```python
from build123d import *

# Parameters (mm, degrees)
F0_R     = 2.89
F0_R_2   = 2.35
F1_DEPTH = 0.81
F0_R_3   = 1.85
F2_DEPTH = 7.885
F3_DEPTH = 0.05


with BuildPart() as f1:
    # F0 (on Front) → F1 (new body, symmetric)
    with BuildSketch(Plane.XZ):
        Circle(F0_R)
        Circle(F0_R_2, mode=Mode.SUBTRACT)
    extrude(amount=F1_DEPTH, both=True)

    # F0 (on Front) → F2 (join, symmetric)
    with BuildSketch(Plane.XZ):
        Circle(F0_R_2)
        Circle(F0_R_3, mode=Mode.SUBTRACT)
    extrude(amount=F2_DEPTH, both=True)

    # F0 (on Front) → F3 (join, symmetric)
    with BuildSketch(Plane.XZ):
        Circle(F0_R_3)
    extrude(amount=F3_DEPTH, both=True)


solid = f1.part
```
Geometry: final body of the model. Coordinates: model frame, mm. A direction names the side the tool comes from. Coordinates: 2 decimals unless noted, no trailing zeros. Write each loop counter-clockwise with the first axis right and the second up, starting at its lowest first coordinate (ties: lowest second). Pieces come first, ordered by that corner, then holes. Notation, with made-up numbers: M 4.5,41 L 48.5,41 A23 cw 48.5,73 Z; hole C 68.5,-24.5 d3. An arc over 180 degrees is marked long. Use CSV: the item, a comma, the result in double quotes. Start each with the question number.
1. Reachability of faces 1 (the face through (-0.401, -3.913, -1.806)), 2 (the face through (-2.29, -0.01, -1.76)), 3 (the face through (-0.509, 4.298, -2.294)) from +Z, -Z, +X, -X, +Y, -Y: full face, straight path, thin tool, end or side. Return the list, or none.
2. First-contact query: P1, Ø2, axis at x = 0, z = 0, coming from the +Y side; P2, Ø1, axis at x = 0, y = 2, coming from the +Z side. Flat tips, straight axial feed; report the tip coordinate or a pass-through.
3. Cut plane D-D on y = 7. Return the cut outline in (x, z).
4. Mould query, pull axis Z, two halves, no side actions, for faces 4 (the face through (-0.509, -4.397, -2.294)), 5 (the face through (-0.401, 4.022, -1.806)). Classes: pulls with the +Z half, pulls with the -Z half, needs draft (parallel to the pull), parting line crosses it, or undercut.
5. Cut plane B-B on x = 0. Return the cut outline in (y, z) (3 decimals).
6. Cut plane C-C on y = -0.25. Return the cut outline in (x, z).
7. Cut plane A-A on z = 0. Return the cut outline in (x, y) (3 decimals).
8. Ray query, probe 1 along Z at (x, y) = (0, 3.75); probe 2 along X at (y, z) = (-5.5, 0.25); probe 3 along Z at (x, y) = (1.7, -4). Return the intervals inside material, ascending.
Entries:
1,face 1,"-Y"
1,face 2,"+Y, -Y"
1,face 3,"+Y"
2,P1,"y = 0.05"
2,P2,"z = 2.35"
3,outline,"C 0,0 d4.7; hole C 0,0 d3.7"
4,face 4,"parting line crosses it"
4,face 5,"undercut"
5,outline,"M -7.885,-2.35 L -0.81,-2.35 L -0.81,-2.89 L 0.81,-2.89 L 0.81,-2.35 L 7.885,-2.35 L 7.885,-1.85 L 0.05,-1.85 L 0.05,1.85 L 7.885,1.85 L 7.885,2.35 L 0.81,2.35 L 0.81,2.89 L -0.81,2.89 L -0.81,2.35 L -7.885,2.35 L -7.885,1.85 L -0.05,1.85 L -0.05,-1.85 L -7.885,-1.85 Z"
6,outline,"C 0,0 d5.78; hole C 0,0 d3.7"
7,outline,"M -2.89,-0.81 L -2.35,-0.81 L -2.35,-7.885 L -1.85,-7.885 L -1.85,-0.05 L 1.85,-0.05 L 1.85,-7.885 L 2.35,-7.885 L 2.35,-0.81 L 2.89,-0.81 L 2.89,0.81 L 2.35,0.81 L 2.35,7.885 L 1.85,7.885 L 1.85,0.05 L -1.85,0.05 L -1.85,7.885 L -2.35,7.885 L -2.35,0.81 L -2.89,0.81 Z"
8,probe 1,"-2.35 to -1.85, 1.85 to 2.35"
8,probe 2,"-2.34 to -1.83, 1.83 to 2.34"
8,probe 3,"-1.62 to -0.73, 0.73 to 1.62"
